Work out the finished part from the listing and answer in its coordinate system (mm). A direction names the side the tool comes from. Round coordinates to 2 decimals unless told otherwise and drop trailing zeros. Loops run counter-clockwise (first coordinate to the right, second up) from the corner with the lowest first, then second, coordinate; pieces in that order, holes last. Notation, with made-up numbers: (36.5, 80) - (71.5, 80) arc R28 ccw to (71.5, 101) - close; hole circle Ø5 at (53.25, 12.25). An arc over 180 degrees is marked (long way). Answer as CSV lines item,"result". Start each with the question number.
Q1. The mould has two halves that part along X. Classify faces 1 (the face through (-32.446, 1.43, 11.191)), 2 (the face through (2, 2.5, 20)), 3 (the face through (-3.08, 3.09, -0.25)), 4 (the face through (-24, 1, 5.056)): +X half, -X half, draft (parallel to the pull), parting line (faces both ways), or undercut.
Q2. Straight lines are drawn through the part: L1, parallel to Y at x = 0, z = -6; L2, parallel to Z at x = -19, y = 1; L3, parallel to Y at x = -30, z = -12. For each, find the intervals that lie inside material, in ascending order. Write a range as [from, to].
Q3. Section D-D on z = -14 is taken. Write down the section's boundary in (x, y).
Q4. For faces 5 (the face through (-24, 1, -4.944)), 6 (the face through (0, 5, -20)), 7 (the face through (2, 2.5, -20)), 8 (the face through (-24, 0, -8)), 9 (the face through (0.51, 2.65, 19.72)), determine the directions among +Z, -Z, +X, -X, +Y, -Y from which every point of the face is accessible in a straight line to the end or side of a thin tool.
Q5. Section A-A on x = -15.5 is taken. Write down the section's boundary in (y, z), then the cut area to 3 significant figures.
Q6. Section C-C on y = 5.75 is taken. Write down the section's boundary in (x, z), then the cut area to 3 significant figures.
Q7. Section B-B on x = -30 is taken. Write down the section's boundary in (y, z).
Q8. Each of these flat-tipped pins is pushed along its axis until it touches: pin 1 Ø8 at (x, z) = (-38, -11) entering from -Y; pin 2 Ø1.6 at (x, y) = (-33, 1.2) entering from -Z; pin 3 Ø3.5 at (y, z) = (6, -19) entering from -X. Where does it stop, or does it pass through?
Autodesk Inventor part; units mm, degrees
ref_plane "YZ Plane" through (0, 0, 0) normal (1, 0, 0) x (0, 1, 0)
ref_plane "XZ Plane" through (0, 0, 0) normal (0, 1, 0) x (-1, 0, 0)
ref_plane "XY Plane" through (0, 0, 0) normal (0, 0, 1) x (1, 0, 0)
sketch "Skizze1" plane through (0, 0, 0) normal (0, 0, 1) x (1, 0, 0)
  line L0 (0, 9.4989) -> (0, -4.4998) construction
  line L1 (-56.1636, 0) -> (12.8813, 0) construction
  circle A0 centre (0, 0) radius 2.5
  arc A1 (-45, 2.5) -> (-45, 0) centre (-45, 1.25) ccw
  line L2 (-45, 2.5) -> (-4.5, 2.5)
  line L3 (-45, 0) -> (-2.5, 0)
  circle A2 centre (0, 0) radius 1.2
  circle A3 centre (-45, 1.2) radius 1.3
  line L4 (0, 2.5) -> (0, 6.9813)
  arc A4 (2.5, 4.4813) -> (0, 6.9813) centre (0, 4.4813) ccw
  line L5 (2.5, 2.5) -> (2.5, 0)
  line L6 (1.0198, 2.5) -> (2.5, 2.5)
  line L7 (2.5, 2.5) -> (2.5, 4.4813)
  arc A5 (0, 6.9813) -> (-2.5, 4.4813) centre (0, 4.4813) ccw
  line L8 (-2.5, 4.4813) -> (-2.5, 4.5)
  arc A6 (-4.5, 2.5) -> (-2.5, 4.5) centre (-4.5, 4.5) ccw
  arc A7 (1.0198, 2.5) -> (0, 2.7) centre (0, 0) ccw
  circle A8 centre (-33, 1.2) radius 0.6
  circle A9 centre (-30, 1.2) radius 0.6
  line L9 (-45, 1.2) -> (0, 1.2) construction
  point P0 (-2.5, 0)
  dimension "d3" = 2.4
  dimension "d0" = 5
  dimension "d1" = 2.5
  dimension "d6" = 45
  dimension "d21" = 2
  dimension "d22" = 0.2
  dimension "d23" = 1.2
  dimension "d24" = 3
  dimension "d25" = 30
extrude "Extrusion1" add sketch "Skizze1" along normal mid plane 35 contours A0 | A0 L4 A7 L6 L5 | A0 L3 A3 L2 A6 A5 L4 | L3 A1 A3 picked at (-45.3896, 1.1022)
extrude "Extrusion6" add sketch "Skizze1" along normal mid plane 44 contours L6 A7 L4 A4 L7
sketch "Skizze2" plane through (-45, 0, 17.5) normal (0, -1, 0) x (1, 0, 0)
  line L0 (8.5763, -17.4438) -> (33.5763, -17.4438) construction
  line L1 (8.5763, -22.4438) -> (33.5763, -22.4438)
  line L2 (33.5763, -12.4438) -> (8.5763, -12.4438)
  arc A0 (8.5763, -12.4438) -> (8.5763, -22.4438) centre (8.5763, -17.4438) ccw
  arc A1 (33.5763, -22.4438) -> (33.5763, -12.4438) centre (33.5763, -17.4438) ccw
  point P0 (45, -17.5)
  point P1 (21.0763, -17.4438)
  dimension "d26" = 10
  dimension "d27" = 25
extrude "Extrusion7" cut sketch "Skizze2" against normal through all
properties part number "Bottom-Lip"
Findings:
1,face 1,"undercut"
1,face 2,"draft"
1,face 3,"-X half"
1,face 4,"undercut"
2,L1,"y = [-2.5, -1.2], [1.2, 6.98]"
2,L2,"z = [-17.5, -4.94], [5.06, 17.5]"
2,L3,"y = [0, 0.6], [1.8, 2.5]"
3,outline,"(-45, 0) - (-2.5, 0) arc R2.5 ccw to (2.5, 0) - (2.5, 4.48) arc R2.5 ccw to (-2.5, 4.48) arc R2 cw to (-4.5, 2.5) - (-45, 2.5) arc R1.25 ccw to start; hole circle Ø1.2 at (-33, 1.2); hole circle Ø1.2 at (-30, 1.2); hole circle Ø2.4 at (0, 0)"
4,face 5,"+Y, -Y"
4,face 6,"-Z, -X, +Y, -Y"
4,face 7,"-Z, +X, -X, -Y"
4,face 8,"+Z, -Z, -X, -Y"
4,face 9,"+Z, -X, -Y"
5,outline,"(0, -17.5) - (2.5, -17.5) - (2.5, -4.94) - (0, -4.94) - close; (0, 5.06) - (2.5, 5.06) - (2.5, 17.5) - (0, 17.5) - close"
5,area,"62.5 mm^2"
6,outline,"(-2.15, -17.5) - (0, -17.5) - (0, -22) - (2.15, -22) - (2.15, 22) - (0, 22) - (0, 17.5) - (-2.15, 17.5) - close"
6,area,"170 mm^2"
7,outline,"(0, -17.5) - (0.6, -17.5) - (0.6, -4.94) - (0, -4.94) - close; (0, 5.06) - (0.6, 5.06) - (0.6, 17.5) - (0, 17.5) - close; (1.8, -17.5) - (2.5, -17.5) - (2.5, -4.94) - (1.8, -4.94) - close; (1.8, 5.06) - (2.5, 5.06) - (2.5, 17.5) - (1.8, 17.5) - close"
8,pin 1,"stops at y = 0"
8,pin 2,"stops at z = -17.5"
8,pin 3,"stops at x = -2.42"
